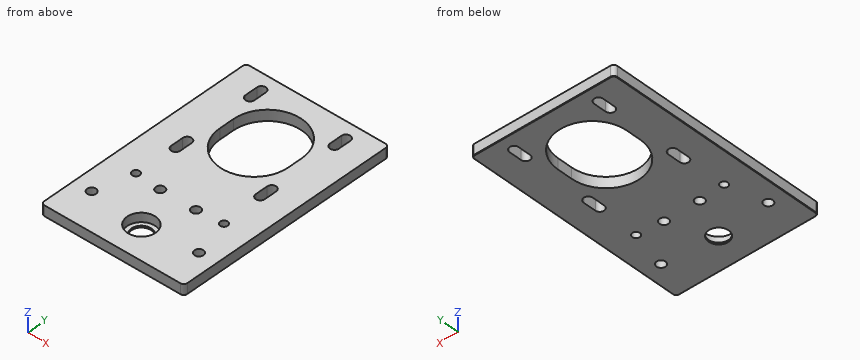
from build123d import *

# Parameters (mm, degrees)
F0_W     = 80
F0_H     = 125
F0_R     = 2.5
F0_R_2   = 2.1
F0_R_3   = 5.59
F1_DEPTH = 6
F3_DEPTH = 6
F4_R     = 2
F5_SIZE  = 0.25
F6_R     = 7.925
F6_R_2   = 5.59
F7_DEPTH = 5


with BuildPart() as f1:
    # F0 (on Top) → F1 (new body)
    with BuildSketch(Plane.XY):
        with Locations((0, 42.5)):
            Rectangle(F0_W, F0_H)
        with Locations((-30, 0)):
            Circle(F0_R, mode=Mode.SUBTRACT)
        with Locations((-24.6, 21.1)):
            Circle(F0_R_2, mode=Mode.SUBTRACT)
        with Locations((-10, 20)):
            Circle(F0_R, mode=Mode.SUBTRACT)
        with Locations((0, -2.4)):
            Circle(F0_R_3, mode=Mode.SUBTRACT)
        with Locations((30, 0)):
            Circle(F0_R, mode=Mode.SUBTRACT)
        with Locations((10, 20)):
            Circle(F0_R, mode=Mode.SUBTRACT)
        with Locations((24.6, 21.1)):
            Circle(F0_R_2, mode=Mode.SUBTRACT)
        with BuildLine():
            ThreePointArc((-19.125, 74.575), (0, 93.7), (19.125, 74.575))
            Line((19.125, 74.575), (19.125, 66.325))
            ThreePointArc((19.125, 66.325), (0, 47.2), (-19.125, 66.325))
            Line((-19.125, 66.325), (-19.125, 74.575))
        make_face(mode=Mode.SUBTRACT)
    extrude(amount=F1_DEPTH)

    # F2 (on Top) → F3 (cut, through all)
    with BuildSketch(Plane.XY):
        with BuildLine():
            Line((-21.125, 89.575), (-21.125, 96.575))
            ThreePointArc((-21.125, 96.575), (-23.625, 99.075), (-26.125, 96.575))
            Line((-26.125, 96.575), (-26.125, 89.575))
            ThreePointArc((-26.125, 89.575), (-23.625, 87.075), (-21.125, 89.575))
        make_face()
        with BuildLine():
            Line((26.125, 89.575), (26.125, 96.575))
            ThreePointArc((26.125, 96.575), (23.625, 99.075), (21.125, 96.575))
            Line((21.125, 96.575), (21.125, 89.575))
            ThreePointArc((21.125, 89.575), (23.625, 87.075), (26.125, 89.575))
        make_face()
        with BuildLine():
            ThreePointArc((21.125, 44.325), (23.625, 41.825), (26.125, 44.325))
            Line((26.125, 44.325), (26.125, 51.325))
            ThreePointArc((26.125, 51.325), (23.625, 53.825), (21.125, 51.325))
            Line((21.125, 51.325), (21.125, 44.325))
        make_face()
        with BuildLine():
            ThreePointArc((-21.125, 51.325), (-23.625, 53.825), (-26.125, 51.325))
            Line((-26.125, 51.325), (-26.125, 44.325))
            ThreePointArc((-26.125, 44.325), (-23.625, 41.825), (-21.125, 44.325))
            Line((-21.125, 44.325), (-21.125, 51.325))
        make_face()
    extrude(amount=F3_DEPTH, mode=Mode.SUBTRACT)

    # F4
    f4_edges = [f1.edges().sort_by_distance(p)[0] for p in [
        (40, -20, 3),
        (-40, -20, 3),
        (40, 105, 3),
        (-40, 105, 3),
    ]]
    fillet(f4_edges, radius=F4_R)

    # F5
    f5_edges = [f1.edges().sort_by_distance(p)[0] for p in [
        (-40, 42.5, 0),
        (-39.414214, 104.414214, 0),
        (0, 105, 0),
        (39.414214, 104.414214, 0),
        (40, 42.5, 0),
        (39.414214, -19.414214, 0),
        (0, -20, 0),
        (-39.414214, -19.414214, 0),
    ]]
    chamfer(f5_edges, length=F5_SIZE)

    # F6 (on face) → F7 (cut)
    with BuildSketch(Plane.XY.offset(6)):
        with Locations((0, -2.4)):
            Circle(F6_R)
        with Locations((0, -2.4)):
            Circle(F6_R_2, mode=Mode.SUBTRACT)
    extrude(amount=-F7_DEPTH, mode=Mode.SUBTRACT)


solid = f1.part
Model file for the job. Use its own axes, mm. Give positions to 0.01 mm unless a question says otherwise; leave off trailing zeros. Loops run counter-clockwise (first coordinate to the right, second up) from the corner with the lowest first, then second, coordinate; pieces in that order, holes last.
1) Wall check: line 1 (X direction, y = 66, z = 1.75); line 2 (X direction, y = 53, z = 4.25); line 3 (Y direction, x = -23, z = 4). Give the ranges that are in metal, low to high.
2) Saw through at D-D (z = 3.5). Count the separate pieces of the cut face and the enclosed holes in it, plus the area to 3 significant figures.
3) Saw through at B-B (y = 82). Write the cut outline in (x, z).
4) Saw through at A-A (x = 30). Write the cut outline in (y, z), plus the area to 3 significant figures.
5) Saw through at C-C (x = 11). Write the cut outline in (y, z).
Answer block:
1. line 1: x = -40 to -19.12, 19.12 to 40
1. line 2: x = -40 to -25.48, -21.77 to -13.72, 13.72 to 21.77, 25.48 to 40
1. line 3: y = -20 to 19.74, 22.46 to 41.9, 53.75 to 87.15, 99 to 105
2. separate pieces: 1
2. enclosed holes: 12
2. area: 8,010 mm2
3. outline: (-40, 0.25) - (-39.75, 0) - (-17.62, 0) - (-17.62, 6) - (-40, 6) - close; (17.62, 0) - (39.75, 0) - (40, 0.25) - (40, 6) - (17.62, 6) - close
4. outline: (-20, 0.25) - (-19.75, 0) - (-2.5, 0) - (-2.5, 6) - (-20, 6) - close; (2.5, 0) - (104.75, 0) - (105, 0.25) - (105, 6) - (2.5, 6) - close
4. area: 720 mm2
5. outline: (-20, 0.25) - (-19.75, 0) - (17.71, 0) - (17.71, 6) - (-20, 6) - close; (22.29, 0) - (50.68, 0) - (50.68, 6) - (22.29, 6) - close; (90.22, 0) - (104.75, 0) - (105, 0.25) - (105, 6) - (90.22, 6) - close
